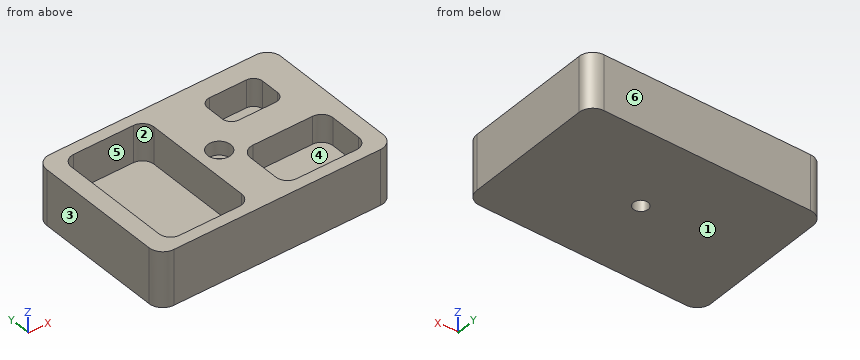
```python
from build123d import *

# Parameters (mm, degrees)
SKETCH1_W                                        = 161.925
SKETCH1_H                                        = 107.95
BOSS_EXTRUDE1_DEPTH                              = 38.1
SKETCH2_W                                        = 57.15
SKETCH2_H                                        = 92.075
CUT_EXTRUDE1_DEPTH                               = 25.4
FILLET1_R                                        = 7.9375
SKETCH3_W                                        = 57.15
SKETCH3_H                                        = 38.1
SKETCH3_W_2                                      = 38.1
SKETCH3_H_2                                      = 25.4
CUT_EXTRUDE2_DEPTH                               = 19.05
FILLET2_R                                        = 6.35
FILLET3_R                                        = 7.9375
FILLET4_R                                        = 9.525
CBORE_FOR_3_8_SOCKET_HEAD_CAP_SCREW1_D           = 10.0838
CBORE_FOR_3_8_SOCKET_HEAD_CAP_SCREW1_CBORE_D     = 15.875
CBORE_FOR_3_8_SOCKET_HEAD_CAP_SCREW1_CBORE_DEPTH = 9.525


with BuildPart() as part:
    # Sketch1 → Boss-Extrude1 (new body)
    with BuildSketch(Plane.XY):
        Rectangle(SKETCH1_W, SKETCH1_H)
    extrude(amount=-BOSS_EXTRUDE1_DEPTH)

    # Sketch2 → Cut-Extrude1 (cut)
    with BuildSketch(Plane.XY):
        with Locations((-40.48125, 0)):
            Rectangle(SKETCH2_W, SKETCH2_H)
    extrude(amount=-CUT_EXTRUDE1_DEPTH, mode=Mode.SUBTRACT)

    # Fillet1
    fillet1_edges = [part.edges().sort_by_distance(p)[0] for p in [
        (-11.90625, 46.0375, -12.7),
        (-11.90625, -46.0375, -12.7),
        (-69.05625, -46.0375, -12.7),
        (-69.05625, 46.0375, -12.7),
    ]]
    fillet(fillet1_edges, radius=FILLET1_R)

    # Sketch3 → Cut-Extrude2 (cut)
    with BuildSketch(Plane.XY):
        with Locations((40.48125, -26.9875)):
            Rectangle(SKETCH3_W, SKETCH3_H)
        with Locations((40.48125, 26.9875)):
            Rectangle(SKETCH3_W_2, SKETCH3_H_2)
    extrude(amount=-CUT_EXTRUDE2_DEPTH, mode=Mode.SUBTRACT)

    # Fillet2
    fillet2_edges = [part.edges().sort_by_distance(p)[0] for p in [
        (59.53125, 39.6875, -9.525),
        (59.53125, 14.2875, -9.525),
        (21.43125, 14.2875, -9.525),
        (21.43125, 39.6875, -9.525),
    ]]
    fillet(fillet2_edges, radius=FILLET2_R)

    # Fillet3
    fillet3_edges = [part.edges().sort_by_distance(p)[0] for p in [
        (69.05625, -7.9375, -9.525),
        (69.05625, -46.0375, -9.525),
        (11.90625, -46.0375, -9.525),
        (11.90625, -7.9375, -9.525),
    ]]
    fillet(fillet3_edges, radius=FILLET3_R)

    # Fillet4
    fillet4_edges = [part.edges().sort_by_distance(p)[0] for p in [
        (80.9625, -53.975, -19.05),
        (-80.9625, -53.975, -19.05),
        (-80.9625, 53.975, -19.05),
        (80.9625, 53.975, -19.05),
    ]]
    fillet(fillet4_edges, radius=FILLET4_R)

    # CBORE for 3/8 Socket Head Cap Screw1 (through all)
    with Locations(Plane.XY):
        with Locations((2.910260727, 0)):
            CounterBoreHole(CBORE_FOR_3_8_SOCKET_HEAD_CAP_SCREW1_D / 2, CBORE_FOR_3_8_SOCKET_HEAD_CAP_SCREW1_CBORE_D / 2, CBORE_FOR_3_8_SOCKET_HEAD_CAP_SCREW1_CBORE_DEPTH)


solid = part.part
```
Can you work these out from the model? Positions are in its coordinate system, mm. Face numbers are marked on the shaded views. A direction names the side the tool comes from. Coordinates: 2 decimals unless noted, no trailing zeros. Loops run counter-clockwise (first coordinate to the right, second up) from the corner with the lowest first, then second, coordinate; pieces in that order, holes last. Notation, with made-up numbers: (1, 24) - (23, 24) arc R8 ccw to (23, 31) - close; hole circle Ø7 at (50.25, -19.75). An arc over 180 degrees is marked (long way). Answer as CSV lines item,"result". Start each with the question number.
1) Which directions (+Z, -Z, +X, -X, +Y, -Y) give clear straight access to the entire face, cutting with the end or side of a thin tool? Please do the marked faces 1 and 2.
2) Suppose I cut it at A-A (y = 0). Please give me the cut outline in (x, z) (1 decimal).
3) Suppose I cut it at B-B (z = -13). Count the separate pieces of the cut face and the enclosed holes in it, plus the area to 3 significant figures.
4) I need wall thicknesses on line 1 (Y direction, x = 46.5, z = -1.5) (1 decimal); line 2 (Y direction, x = -38.5, z = -22.5) (1 decimal); line 3 (Y direction, x = 3.5, z = -2) (3 decimals). Which ranges of each line are inside material? Lowest first, please. Write a range as from..to.
5) Thinking about a two-plate mould opening in X: for the marked faces 3, 4, 5 and 6, which applies, pulls with the +X half, pulls with the -X half, needs draft (parallel to the pull), parting line crosses it, or undercut?
6) Suppose I cut it at C-C (x = -57). Please give me the cut outline in (y, z) (1 decimal).
7) For pin 1 (17 mm diameter, centred on x = -48.5, y = -10.5, fed in from +Z); pin 2 (14.5 mm diameter, centred on x = 2.91, y = 0, fed in from +Z) (3 decimals); pin 3 (12.5 mm diameter, centred on x = 47.5, y = 29.5, fed in from +Z); pin 4 (9 mm diameter, centred on x = 2.91, y = 0, fed in from +Z), each with a flat end and sliding along its axis, tell me the tip position at first contact or that it passes through.
Check result:
1,face 1,"-Z, +X, -X, +Y, -Y"
1,face 2,"+Z"
2,outline,"(-81, -38.1) - (-2.1, -38.1) - (-2.1, -9.5) - (-5, -9.5) - (-5, 0) - (-11.9, 0) - (-11.9, -25.4) - (-69.1, -25.4) - (-69.1, 0) - (-81, 0) - close; (8, -38.1) - (81, -38.1) - (81, 0) - (10.8, 0) - (10.8, -9.5) - (8, -9.5) - close"
3,separate pieces,"1"
3,enclosed holes,"4"
3,area,"9,060 mm²"
4,line 1,"y = -54..-46, -7.9..14.3, 39.7..54"
4,line 2,"y = -54..-46, 46..54"
4,line 3,"y = -53.975..-7.916, 7.916..53.975"
5,face 3,"pulls with the -X half"
5,face 4,"undercut"
5,face 5,"undercut"
5,face 6,"needs draft"
6,outline,"(-54, -38.1) - (54, -38.1) - (54, 0) - (46, 0) - (46, -25.4) - (-46, -25.4) - (-46, 0) - (-54, 0) - close"
7,pin 1,"stops at z = -25.4"
7,pin 2,"stops at z = -9.525"
7,pin 3,"stops at z = -19.05"
7,pin 4,"passes through"
